Could you check a few things on this model? Use its own coordinates, in mm. Give positions to 0.01 mm unless a question says otherwise; leave off trailing zeros. Order: outer loops, then holes, each group sorted by start corner. A loop starts at its lowest first (then second) coordinate and runs counter-clockwise, first axis right, second up. Notation, with made-up numbers: (61.5, 33) - (116.5, 33) arc R18 cw to (116.5, 68) - close; hole circle Ø6 at (-11.75, -16.5). An arc over 180 degrees is marked (long way). One line per question, with ' | ' between items. Start each with the question number.
1. Imagine slicing it at A-A (y = 0). Please give me the cut outline in (x, z).
2. I need wall thicknesses on probe 1 along Y at (x, z) = (0, -0.5); probe 2 along X at (y, z) = (4.5, -1.25); probe 3 along X at (y, z) = (9, -1.75). Which ranges of each line are inside material? Lowest first, please. Write a range as from..to.
3. Imagine slicing it at D-D (y = -23.5). Please give me the cut outline in (x, z), and give its area (3 significant figures).
4. Imagine slicing it at B-B (x = -4.5). Please give me the cut outline in (y, z), and give its area (3 significant figures).
5. Imagine slicing it at C-C (z = -2.75). Please give me the cut outline in (x, y), and give its area (3 significant figures).
6. If we mould it in two halves opening along X, with no side actions, what happens to faces 1 (the flat face through (74, 30, 0)), 2 (the cylindrical face through (-29.993, -0.66, -0.07)), 3 (the cylindrical face through (139, 0, 0)), 4 (the cylindrical face through (-2.38, 10.74, -0.07))? For each: released by +X, released by -X, zero draft, split by the parting line, or undercut.
7. For P1, Ø2, axis at x = 151.5, z = -3.5, coming from the +Y side; P2, Ø1, axis at y = 23.5, z = 1.5, coming from the +X side; P3, Ø17.5, axis at x = 0, y = 0, coming from the -Z side; P4, Ø1.5, axis at y = 9, z = 0.5, coming from the -X side, each with a flat end and sliding along its axis, tell me the tip position at first contact or that it passes through.
Autodesk Inventor part; units mm, degrees
ref_plane "YZ Plane" through (0, 0, 0) normal (1, 0, 0) x (0, 1, 0)
ref_plane "XZ Plane" through (0, 0, 0) normal (0, 1, 0) x (-1, 0, 0)
ref_plane "XY Plane" through (0, 0, 0) normal (0, 0, 1) x (1, 0, 0)
sketch "Sketch1" plane through (0, 0, 0) normal (0, 0, 1) x (1, 0, 0)
  circle A0 centre (0, 0) radius 11
  arc A1 (0, 30) -> (0, -30) centre (0, 0) ccw
  line L0 (0, 30) -> (150, 30)
  circle A2 centre (150, 0) radius 11
  line L1 (0, -30) -> (150, -30)
  arc A3 (150, -30) -> (150, 30) centre (150, 0) ccw
  dimension "d0" = 22
  dimension "d1" = 30
  dimension "d2" = 150
  dimension "d3" = 22
  dimension "d6" = 150
extrude "Extrusion1" add sketch "Sketch1" along normal mid plane 10
equation "\"d6\" = d2"
properties part number "Suporte"
Results found:
1) outline: (-30, -5) - (-11, -5) - (-11, 5) - (-30, 5) - close; (11, -5) - (139, -5) - (139, 5) - (11, 5) - close; (161, -5) - (180, -5) - (180, 5) - (161, 5) - close
2) probe 1: y = -30..-11, 11..30 | probe 2: x = -29.66..-10.04, 10.04..139.96, 160.04..179.66 | probe 3: x = -28.62..-6.32, 6.32..143.68, 156.32..178.62
3) outline: (-18.65, -5) - (168.65, -5) - (168.65, 5) - (-18.65, 5) - close | area: 1,870 mm2
4) outline: (-29.66, -5) - (-10.04, -5) - (-10.04, 5) - (-29.66, 5) - close; (10.04, -5) - (29.66, -5) - (29.66, 5) - (10.04, 5) - close | area: 392 mm2
5) outline: (0, -30) - (150, -30) arc R30 ccw to (150, 30) - (0, 30) arc R30 ccw to start; hole circle Ø22 at (0, 0); hole circle Ø22 at (150, 0) | area: 11,100 mm2
6) face 1: zero draft | face 2: released by -X | face 3: undercut | face 4: undercut
7) P1: stops at y = 30 | P2: stops at x = 169.26 | P3: passes through | P4: stops at x = -28.84
